Work out the finished part from the listing and answer in its coordinate system (mm). A direction names the side the tool comes from. Give positions to 0.01 mm unless a question says otherwise; leave off trailing zeros. Loops run counter-clockwise (first coordinate to the right, second up) from the corner with the lowest first, then second, coordinate; pieces in that order, holes last.
from build123d import *

# Parameters (mm, degrees)
F0_W     = 50.8
F0_H     = 50.8
F1_DEPTH = 74.6125
F3_D     = 22.225
F3_DEPTH = 57.15
F3_TIP   = 6.6770636289


with BuildPart() as f1:
    # F0 (on Top) → F1 (new body, symmetric)
    with BuildSketch(Plane.XY):
        Rectangle(F0_W, F0_H)
    extrude(amount=F1_DEPTH, both=True)

    # F3
    with Locations(Plane.XY.offset(74.6125)):
        with Locations((0, 0)):
            Hole(F3_D / 2, depth=F3_DEPTH)
            with Locations((0, 0, -(F3_DEPTH + F3_TIP / 2))):  # 118° drill point
                Cone(0, F3_D / 2, F3_TIP, mode=Mode.SUBTRACT)


solid = f1.part
Item 1: Consider line 1 (X direction, y = 0, z = 44.5); line 2 (Y direction, x = 0.5, z = 26); line 3 (Y direction, x = -7, z = 66.5). Determine where each line is inside the solid, lowest interval first.
Item 2: For faces 1 (the face through (0, 0, -74.612)), 2 (the face through (-10.6, 3.34, 45.64)), determine the directions among +Z, -Z, +X, -X, +Y, -Y from which every point of the face is accessible in a straight line to the end or side of a thin tool.
Item 3: Determine the mould class of faces 3 (the face through (0, 12, 74.612)), 4 (the face through (-0.418, -1.884, 11.945)), 5 (the face through (0, 25.4, 1)) for opening direction Y: released by +Y, released by -Y, zero draft, split by the parting line, or undercut.
Item 4: Find section A-A, the plane z = 30.5. Write down the section's boundary in (x, y) (1 decimal), plus the area to 3 significant figures.
Ans:
1. line 1: x = -25.4 to -11.11, 11.11 to 25.4
1. line 2: y = -25.4 to -11.1, 11.1 to 25.4
1. line 3: y = -25.4 to -8.63, 8.63 to 25.4
2. face 1: -Z, +X, -X, +Y, -Y
2. face 2: +Z
3. face 3: zero draft
3. face 4: undercut
3. face 5: released by +Y
4. outline: (-25.4, -25.4) - (25.4, -25.4) - (25.4, 25.4) - (-25.4, 25.4) - close; hole circle Ø22.2 at (0, 0)
4. area: 2,190 mm2
